Model file for the job. Use its own axes, mm. A direction names the side the tool comes from. Round coordinates to 2 decimals unless told otherwise and drop trailing zeros. Return JSON: item names as keys, results as strings. Group by question number.
Item 1: Pull direction X, two halves, no side cores. Call faces 6 (the face through (21.65, 4.16, 6.4)), 7 (the face through (-21.39, 2.02, 6.4)), 8 (the face through (5.94, 39.32, 3.45)): pulls with the +X half, pulls with the -X half, needs draft (parallel to the pull), parting line crosses it, or undercut.
Item 2: Slice it at A-A on y = -9. Give the number of separate pieces and of enclosed holes in the cut face, then the cut area to 3 significant figures.
Item 3: Which spindle directions (+Z, -Z, +X, -X, +Y, -Y) get a long thin tool onto all of the face, cutting with end or side? Do faces 1 (the face through (-7.843, -21.849, 3.479)), 2 (the face through (8.94, -19.53, 6.4)), 3 (the face through (-12, 15, 3)), 4 (the face through (-14.43, 16.67, 0.6)), 5 (the face through (-6, -11, 0)). Say none if no direction does.
Item 4: Pin check, flat tips, straight feed: pin 1 Ø1.5 at (y, z) = (2, 2) entering from +X; pin 2 Ø3.5 at (y, z) = (12, 3.5) entering from -X; pin 3 Ø2 at (x, z) = (19, 1.5) entering from +Y. Stop position of each tip, or through.
Item 5: Probe line 1 along Y through (x, z) = (17, 4.75); line 2 along X through (y, z) = (-3, 3); line 3 along Y through (x, z) = (5.5, 0.5). List the from-to ranges inside material, lowest first.
from build123d import *

# Parameters (mm, degrees)
F0_R     = 11.05
F1_DEPTH = 7
F2_R     = 2


with BuildPart() as f1:
    # F0 (on Top) → F1 (new body)
    with BuildSketch(Plane.XY):
        with BuildLine():
            ThreePointArc((7.5, 12.9903810568), (11.2230439167, 9.9520492987), (13.7942286341, 5.8923048454))
            Line((13.7942286341, 5.8923048454), (24.1865334795, -0.1076951546))
            ThreePointArc((24.1865334795, -0.1076951546), (28.9879676676, -0.304534211), (33.4807621135, -2.0096189432))
            Line((33.4807621135, -2.0096189432), (11.903289687, 10.4481405707))
            Line((11.903289687, 10.4481405707), (7.5, 12.9903810568))
        make_face()
        with BuildLine():
            ThreePointArc((14.8335897314, -25.0369590954), (11.0629336807, -16.5679269269), (12.990381079, -7.4999999614))
            ThreePointArc((12.990381079, -7.4999999614), (10.6066017336, -10.606601702), (7.5, -12.9903810568))
            Line((7.5, -12.9903810568), (3.096710313, -15.5326215429))
            Line((3.096710313, -15.5326215429), (14.8335897314, -25.0369590954))
        make_face()
        with BuildLine():
            ThreePointArc((24.1865334795, -0.1076951546), (17.7159140598, -2.4823210359), (12.990381079, -7.4999999614))
            ThreePointArc((12.990381079, -7.4999999614), (11.0629336807, -16.5679269269), (14.8335897314, -25.0369590954))
            Line((14.8335897314, -25.0369590954), (18.4807621135, -27.9903810568))
            ThreePointArc((18.4807621135, -27.9903810568), (33.4807621135, -27.9903810568), (40.9807621135, -15))
            ThreePointArc((40.9807621135, -15), (38.9711431703, -7.5), (33.4807621135, -2.0096189432))
            ThreePointArc((33.4807621135, -2.0096189432), (28.9879676676, -0.304534211), (24.1865334795, -0.1076951546))
        make_face()
        with Locations((25.9807621135, -15)):
            Circle(F0_R, mode=Mode.SUBTRACT)
        with BuildLine():
            ThreePointArc((0, 15), (3.8822856765, 14.4888873943), (7.5, 12.9903810568))
            Line((7.5, 12.9903810568), (11.903289687, 10.4481405707))
            Line((11.903289687, 10.4481405707), (14.2658477444, 25.3647450844))
            ThreePointArc((14.2658477444, 25.3647450844), (8.8167787844, 17.8647450844), (0, 15))
        make_face()
        with BuildLine():
            Line((3.096710313, -15.5326215429), (7.5, -12.9903810568))
            ThreePointArc((7.5, -12.9903810568), (3.0072055541, -14.695465789), (-1.7942286341, -14.8923048454))
            Line((-1.7942286341, -14.8923048454), (-12.1865334795, -20.8923048454))
            ThreePointArc((-12.1865334795, -20.8923048454), (-14.7577181969, -24.9520492987), (-18.4807621135, -27.9903810568))
            Line((-18.4807621135, -27.9903810568), (3.096710313, -15.5326215429))
        make_face()
        with BuildLine():
            Line((18.4807621135, -27.9903810568), (14.8335897314, -25.0369590954))
            ThreePointArc((14.8335897314, -25.0369590954), (16.5409562478, -26.6571894219), (18.4807621135, -27.9903810568))
        make_face()
        with BuildLine():
            ThreePointArc((-12, 21), (-6.7082039325, 16.583592135), (0, 15))
            ThreePointArc((0, 15), (8.8167787844, 17.8647450844), (14.2658477444, 25.3647450844))
            Line((14.2658477444, 25.3647450844), (15, 30))
            ThreePointArc((15, 30), (0, 45), (-15, 30))
            ThreePointArc((-15, 30), (-14.2302494708, 25.2565835097), (-12, 21))
        make_face()
        with Locations((0, 30)):
            Circle(F0_R, mode=Mode.SUBTRACT)
        with BuildLine():
            ThreePointArc((-15, 0), (-14.2302494708, 4.7434164903), (-12, 9))
            Line((-12, 9), (-12, 21))
            ThreePointArc((-12, 21), (-14.2302494708, 25.2565835097), (-15, 30))
            Line((-15, 30), (-15, 5.0844809722))
            Line((-15, 5.0844809722), (-15, 0))
        make_face()
        with BuildLine():
            Line((15, 30), (14.2658477444, 25.3647450844))
            ThreePointArc((14.2658477444, 25.3647450844), (14.8153251089, 27.6534830244), (15, 30))
        make_face()
        with BuildLine():
            ThreePointArc((-29.0994374758, -0.327785989), (-19.8797124097, -1.2968181611), (-12.9903809936, -7.5000001095))
            ThreePointArc((-12.9903809936, -7.5000001095), (-14.488887378, -3.8822857376), (-15, 0))
            Line((-15, 0), (-15, 5.0844809722))
            Line((-15, 5.0844809722), (-29.0994374758, -0.327785989))
        make_face()
        with BuildLine():
            ThreePointArc((-10.9807621135, -15), (-11.4918747028, -11.1177143845), (-12.9903809936, -7.5000001095))
            ThreePointArc((-12.9903809936, -7.5000001095), (-19.8797124097, -1.2968181611), (-29.0994374758, -0.327785989))
            Line((-29.0994374758, -0.327785989), (-33.4807621135, -2.0096189432))
            ThreePointArc((-33.4807621135, -2.0096189432), (-38.9711431703, -22.5), (-18.4807621135, -27.9903810568))
            ThreePointArc((-18.4807621135, -27.9903810568), (-14.7577181969, -24.9520492987), (-12.1865334795, -20.8923048454))
            ThreePointArc((-12.1865334795, -20.8923048454), (-11.2852963245, -18.0072055541), (-10.9807621135, -15))
        make_face()
        with Locations((-25.9807621135, -15)):
            Circle(F0_R, mode=Mode.SUBTRACT)
        with BuildLine():
            Line((-33.4807621135, -2.0096189432), (-29.0994374758, -0.327785989))
            ThreePointArc((-29.0994374758, -0.327785989), (-31.3562813567, -0.9962936025), (-33.4807621135, -2.0096189432))
        make_face()
        with BuildLine():
            ThreePointArc((12.990381079, -7.4999999614), (14.4888874001, -3.882285655), (15, 0))
            ThreePointArc((15, 0), (14.695465789, 3.0072055541), (13.7942286341, 5.8923048454))
            ThreePointArc((13.7942286341, 5.8923048454), (11.2230439167, 9.9520492987), (7.5, 12.9903810568))
            ThreePointArc((7.5, 12.9903810568), (3.8822856765, 14.4888873943), (0, 15))
            ThreePointArc((0, 15), (-6.7082039325, 13.416407865), (-12, 9))
            ThreePointArc((-12, 9), (-14.2302494708, 4.7434164903), (-15, 0))
            ThreePointArc((-15, 0), (-14.488887378, -3.8822857376), (-12.9903809936, -7.5000001095))
            ThreePointArc((-12.9903809936, -7.5000001095), (-8.2648480196, -12.5176789866), (-1.7942286341, -14.8923048454))
            ThreePointArc((-1.7942286341, -14.8923048454), (3.0072055541, -14.695465789), (7.5, -12.9903810568))
            ThreePointArc((7.5, -12.9903810568), (10.6066017336, -10.606601702), (12.990381079, -7.4999999614))
        make_face()
        Circle(F0_R, mode=Mode.SUBTRACT)
    extrude(amount=F1_DEPTH)

    # F2
    f2_edges = [f1.edges().sort_by_distance(p)[0] for p in [
        (22.692026, 4.219261, 0),
        (37.637952, -24.439806, 0),
        (8.96515, -20.28479, 0),
        (-7.692026, -21.761501, 0),
        (-22.049719, 2.378347, 0),
        (-15, 17.54224, 0),
        (13.084569, 17.906443, 0),
        (-15, 17.54224, 7),
        (-22.049719, 2.378347, 7),
        (-7.692026, -21.761501, 7),
        (8.96515, -20.28479, 7),
        (22.692026, 4.219261, 7),
        (13.084569, 17.906443, 7),
    ]]
    fillet(f2_edges, radius=F2_R)


solid = f1.part
Output values:
{
 "1": {"face 6": "pulls with the +X half", "face 7": "pulls with the -X half", "face 8": "undercut"},
 "2": {"separate pieces": "5", "enclosed holes": "0", "area": "201 mm²"},
 "3": {"face 1": "+Z, -Z, -Y", "face 2": "+Z, -Y", "face 3": "+Z, -Z", "face 4": "-Z, -X, +Y", "face 5": "-Z, +X, -X, +Y, -Y"},
 "4": {"pin 1": "x = 27.83", "pin 2": "x = -15", "pin 3": "y = 6.89"},
 "5": {"line 1": "-27.01 to -21.44, -8.56 to -2.99, 4.04 to 7.51", "line 2": "-34.98 to -10.63, 10.63 to 14.7, 16.98 to 34.98", "line 3": "-16.61 to -9.58, 9.58 to 20.42, 39.58 to 43.22"}
}
